For this review, use the dimensioned drawing (mm, ordinates from the lowest corner) and the shaded views. A direction names the side the tool comes from. Give positions to 0.01 mm unless a question says otherwise; leave off trailing zeros. Write each loop counter-clockwise with the first axis right and the second up, starting at its lowest first coordinate (ties: lowest second). Pieces come first, ordered by that corner, then holes. Notation, with made-up numbers: M -17,73.25 L -13,73.25 A22 ccw -13,111.25 Z; hole C 34.5,36.25 d1. An arc over 180 degrees is marked long. Answer in a Markdown table with one row per item.
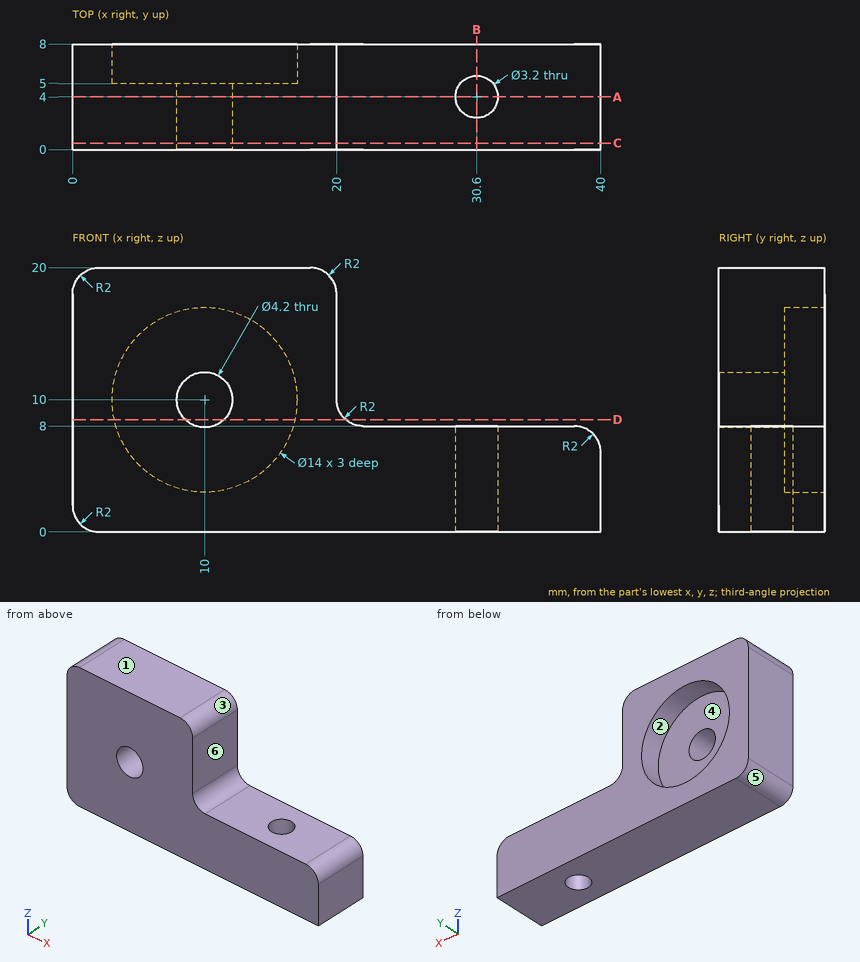
1) The part is to be moulded in two halves that separate along X. For the marked faces 1, 2 and 3, say which applies: released by +X, released by -X, zero draft, split by the parting line, or undercut.
Geometry says:
| item | result |
|---|---|
| face 1 | zero draft |
| face 2 | undercut |
| face 3 | released by +X |
2) Add section B-B (x = 30.6). Write out the cut boundary in (y, z), and give its area (3 significant figures).
Geometry says:
| item | result |
|---|---|
| outline | M 0,0 L 2.4,0 L 2.4,8 L 0,8 Z; M 5.6,0 L 8,0 L 8,8 L 5.6,8 Z |
| area | 38.4 mm^2 |
3) Add section A-A (y = 4). Write out the cut boundary in (x, z), and give its area (3 significant figures).
Geometry says:
| item | result |
|---|---|
| outline | M 0,2 A2 ccw 2,0 L 29,0 L 29,8 L 22,8 A2 cw 20,10 L 20,18 A2 ccw 18,20 L 2,20 A2 ccw 0,18 Z; M 32.2,0 L 40,0 L 40,6 A2 ccw 38,8 L 32.2,8 Z; hole C 10,10 d4.2 |
| area | 518 mm^2 |
4) For the marked faces 4, 5 and 6, list the 3-axis set-ups (+Z, -Z, +X, -X, +Y, -Y) from which the entire face can be reached by the end or side of a thin tool; tool diameter is ignored.
Geometry says:
| item | result |
|---|---|
| face 4 | +Y |
| face 5 | -Z, -X, +Y, -Y |
| face 6 | +Z, +X, +Y, -Y |
5) Insertion check: P1, Ø4, axis at y = 2.5, z = 15, coming from the +X side. The pin has a flat end and moves straight along its axis. Give the tip position at first contact, or say it passes through.
Geometry says:
| item | result |
|---|---|
| P1 | x = 20 |
6) Add section C-C (y = 0.5). Write out the cut boundary in (x, z), and give its area (3 significant figures).
Geometry says:
| item | result |
|---|---|
| outline | M 0,2 A2 ccw 2,0 L 40,0 L 40,6 A2 ccw 38,8 L 22,8 A2 cw 20,10 L 20,18 A2 ccw 18,20 L 2,20 A2 ccw 0,18 Z; hole C 10,10 d4.2 |
| area | 544 mm^2 |
7) Add section D-D (z = 8.5). Write out the cut boundary in (x, y).
Geometry says:
| item | result |
|---|---|
| outline | M 0,0 L 8.53,0 L 8.53,5 L 3.16,5 L 3.16,8 L 0,8 Z; M 11.47,0 L 20.68,0 L 20.68,8 L 16.84,8 L 16.84,5 L 11.47,5 Z |
8) To check wall thickness, follow probe 1 along X at (y, z) = (6.15, 10); probe 2 along Z at (x, y) = (10, 1.4). State the ranges of each line that lie inside material, in increasing order. Write a range as [from, to].
Geometry says:
| item | result |
|---|---|
| probe 1 | [0, 3], [17, 20] |
| probe 2 | [0, 7.9], [12.1, 20] |
